```python
from build123d import *

# Parameters (mm, degrees)
F0_W     = 1203.49264
F0_H     = 448.315588
F1_DEPTH = 25.4
F2_W     = 1316.091538
F2_H     = 697.101116
F3_DEPTH = 25.4
F4_W     = 641.82043
F4_H     = 398.742794
F5_DEPTH = 25.4


with BuildPart() as f1:
    # F0 (on Front) → F1 (new body)
    with BuildSketch(Plane.XZ):
        Rectangle(F0_W, F0_H)
    extrude(amount=F1_DEPTH)

    # F2 (on Top) → F3 (join)
    with BuildSketch(Plane.XY):
        Rectangle(F2_W, F2_H)
    extrude(amount=F3_DEPTH)

    # F4 (on Right) → F5 (join)
    with BuildSketch(Plane.YZ):
        Rectangle(F4_W, F4_H)
    extrude(amount=F5_DEPTH)


solid = f1.part
```
Work out the finished part from the listing and answer in its coordinate system (mm). A direction names the side the tool comes from. Give positions to 0.01 mm unless a question says otherwise; leave off trailing zeros. Order: outer loops, then holes, each group sorted by start corner. A loop starts at its lowest first (then second) coordinate and runs counter-clockwise, first axis right, second up. Notation, with made-up numbers: (-8, 1.5) -> (35, 1.5) arc R6 cw to (35, 5.5) -> close; hole circle Ø7 at (61, 88.25). An arc over 180 degrees is marked (long way). Answer as CSV lines item,"result". Start each with the question number.
(1) Each of these flat-tipped pins is pushed along its axis until it touches: pin 1 Ø8 at (y, z) = (-5, -98.5) entering from +X; pin 2 Ø7.5 at (y, z) = (-18, -115.5) entering from -X; pin 3 Ø12.5 at (x, z) = (11, 97.5) entering from -Y. Where does it stop, or does it pass through?
(2) Section A-A, the plane y = 252.5 is taken. Write down the section's boundary in (x, z).
(3) Consider line 1 along X through (y, z) = (240.5, 182.5); line 2 along Y through (x, z) = (133.5, -156.5). Determine where each line is inside the solid, lowest interval first.
(4) Section B-B, the plane z = -36.5 is taken. Write down the section's boundary in (x, y), plus the area to 3 significant figures.
(5) Which of the six approach directions +Z, -Z, +X, -X, +Y, -Y give full straight-line access (tool end or side, diameter ignored) to faces 1 (the flat face through (13, -175, -199.371)), 2 (the flat face through (-601.746, -13, 123)), 3 (the flat face through (13, 158, 199.371)), 4 (the flat face through (13, -320.91, 111)), 5 (the flat face through (601.746, -13, -114))?
Entries:
1,pin 1,"x = 601.75"
1,pin 2,"x = -601.75"
1,pin 3,"y = -320.91"
2,outline,"(-658.05, 0) -> (0, 0) -> (0, -199.37) -> (25.4, -199.37) -> (25.4, 0) -> (658.05, 0) -> (658.05, 25.4) -> (25.4, 25.4) -> (25.4, 199.37) -> (0, 199.37) -> (0, 25.4) -> (-658.05, 25.4) -> close"
3,line 1,"0 to 25.4"
3,line 2,"-25.4 to 0"
4,outline,"(-601.75, -25.4) -> (0, -25.4) -> (0, -320.91) -> (25.4, -320.91) -> (25.4, -25.4) -> (601.75, -25.4) -> (601.75, 0) -> (25.4, 0) -> (25.4, 320.91) -> (0, 320.91) -> (0, 0) -> (-601.75, 0) -> close"
4,area,"46,200 mm²"
5,face 1,"-Z, +X, -X, -Y"
5,face 2,"+Z, -X, +Y, -Y"
5,face 3,"+Z, +X, -X, +Y"
5,face 4,"+Z, +X, -X, -Y"
5,face 5,"-Z, +X, +Y, -Y"
